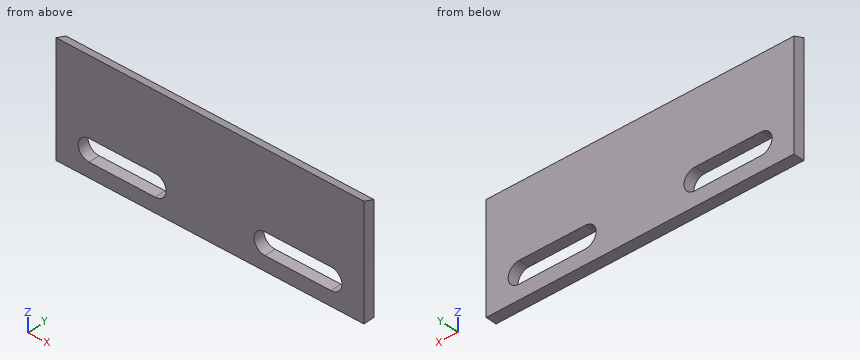
```python
from build123d import *

# Parameters (mm, degrees)
SKETCH1_W           = 533.146
SKETCH1_H           = 196.863399688
BOSS_EXTRUDE1_DEPTH = 19.05
CUT_EXTRUDE1_DEPTH  = 7702.120410186
CUT_EXTRUDE2_DEPTH  = 7008.877833132


with BuildPart() as part:
    # Sketch1 → Boss-Extrude1 (new body)
    with BuildSketch(Plane(origin=(0, 3140.71, 0), x_dir=(1, 0, 0), z_dir=(0, 1, 0))):
        with Locations((0, 6904.348295077)):
            Rectangle(SKETCH1_W, SKETCH1_H)
    extrude(amount=BOSS_EXTRUDE1_DEPTH)

    # Sketch2 → Cut-Extrude1 (cut, through all)
    with BuildSketch(Plane(origin=(266.573, 0, 0), x_dir=(0, 0, -1), z_dir=(1, 0, 0))):
        Polygon((6805.916595233, 3140.710000001), (6813.613294835, 3159.760000001), (6805.916595233, 3159.760000001), align=None)
    extrude(amount=-CUT_EXTRUDE1_DEPTH, mode=Mode.SUBTRACT)

    # Sketch3 → Cut-Extrude2 (cut, through all)
    with BuildSketch(Plane(origin=(0, 3159.76, 0), x_dir=(1, 0, 0), z_dir=(0, 1, 0))):
        with BuildLine():
            Line((209.423, 6939.279994921), (95.123, 6939.279994921))
            ThreePointArc((95.123, 6939.279994921), (76.073, 6958.329994921), (95.123, 6977.379994921))
            Line((95.123, 6977.379994921), (209.423, 6977.379994921))
            ThreePointArc((209.423, 6977.379994921), (228.473, 6958.329994921), (209.423, 6939.279994921))
        make_face()
        with BuildLine():
            Line((-209.423, 6939.279994921), (-95.123, 6939.279994921))
            ThreePointArc((-95.123, 6939.279994921), (-76.073, 6958.329994921), (-95.123, 6977.379994921))
            Line((-95.123, 6977.379994921), (-209.423, 6977.379994921))
            ThreePointArc((-209.423, 6977.379994921), (-228.473, 6958.329994921), (-209.423, 6939.279994921))
        make_face()
    extrude(amount=-CUT_EXTRUDE2_DEPTH, mode=Mode.SUBTRACT)


solid = part.part
```
Read the model definition and answer for the solid it produces. Units are mm, in the model's axes. Coordinates: 2 decimals unless noted, no trailing zeros. Loops run counter-clockwise (first coordinate to the right, second up) from the corner with the lowest first, then second, coordinate; pieces in that order, holes last.
(1) The part is cut by section C-C (y = 3148.25). Determine the outline of the cut face in (x, z), and give its area (3 significant figures).
Solution:
outline: (-266.57, -7002.78) - (266.57, -7002.78) - (266.57, -6808.96) - (-266.57, -6808.96) - close; hole (-209.42, -6977.38) - (-95.12, -6977.38) arc R19.05 ccw to (-95.12, -6939.28) - (-209.42, -6939.28) arc R19.05 ccw to start; hole (95.12, -6977.38) - (209.42, -6977.38) arc R19.05 ccw to (209.42, -6939.28) - (95.12, -6939.28) arc R19.05 ccw to start
area: 92,300 mm2
(2) Consider line 1 along X through (y, z) = (3154.5, -6959); line 2 along X through (y, z) = (3158.25, -6956.5); line 3 along Z through (x, y) = (-142.5, 3147.5). Determine where each line is inside the solid, lowest interval first.
Solution:
line 1: x = -266.57 to -228.46, -76.08 to 76.08, 228.46 to 266.57
line 2: x = -266.57 to -228.38, -76.16 to 76.16, 228.38 to 266.57
line 3: z = -7002.78 to -6977.38, -6939.28 to -6808.66
(3) Flat-ended cylindrical pins translate along their axes: pin 1 Ø5.5 at (x, y) = (-152.5, 3153.5) entering from +Z; pin 2 Ø5.5 at (x, y) = (131, 3153) entering from +Z; pin 3 Ø3 at (x, y) = (-13.5, 3154) entering from +Z. Find the tip coordinate at first contact, or state that the pin passes through.
Solution:
pin 1: stops at z = -6809.97
pin 2: stops at z = -6809.77
pin 3: stops at z = -6810.68
(4) The part is cut by section D-D (x = -32.5). Determine the outline of the cut face in (y, z), and give its area (3 significant figures).
Solution:
outline: (3140.71, -7002.78) - (3159.76, -7002.78) - (3159.76, -6813.61) - (3140.71, -6805.92) - close
area: 3,680 mm2
(5) The part is cut by section A-A (x = 113.5). Determine the outline of the cut face in (y, z), and give its area (3 significant figures).
Solution:
outline: (3140.71, -7002.78) - (3159.76, -7002.78) - (3159.76, -6977.38) - (3140.71, -6977.38) - close; (3140.71, -6939.28) - (3159.76, -6939.28) - (3159.76, -6813.61) - (3140.71, -6805.92) - close
area: 2,950 mm2
(6) The part is cut by section B-B (z = -6950.5). Determine the outline of the cut face in (x, y).
Solution:
outline: (-266.57, 3140.71) - (-226.79, 3140.71) - (-226.79, 3159.76) - (-266.57, 3159.76) - close; (-77.76, 3140.71) - (77.76, 3140.71) - (77.76, 3159.76) - (-77.76, 3159.76) - close; (226.79, 3140.71) - (266.57, 3140.71) - (266.57, 3159.76) - (226.79, 3159.76) - close
